```python
from build123d import *

# Parameters (mm, degrees)
PAD_DEPTH       = 6
SKETCH001_R     = 2
POCKET_DEPTH    = 8
POCKET001_DEPTH = 7


with BuildPart() as part:
    # Sketch → Pad (new body)
    with BuildSketch(Plane.XY):
        Polygon((1, 94.8), (7, 94.8), (7, 10), (8, 10), (8, 0), (0, 0), (0, 10), (1, 10), align=None)
    extrude(amount=PAD_DEPTH)

    # Sketch001 (on Face10 of Pad) → Pocket (cut)
    with BuildSketch(Plane.XY.offset(6)):
        with Locations((4, 4.995998)):
            Circle(SKETCH001_R)
    extrude(amount=-POCKET_DEPTH, mode=Mode.SUBTRACT)

    # Sketch002 (on Face5 of Pocket) → Pocket001 (cut)
    with BuildSketch(Plane.XY.offset(6)):
        with BuildLine():
            ThreePointArc((0, 1), (0.292893, 0.292893), (1, 0))
            Line((0, 0), (1, 0))
            Line((0, 1), (0, 0))
        make_face()
        with BuildLine():
            ThreePointArc((1, 10), (0.292893, 9.707107), (0, 9))
            Line((0, 9), (0, 10))
            Line((0, 10), (1, 10))
        make_face()
        with BuildLine():
            ThreePointArc((8, 9), (7.707107, 9.707107), (7, 10))
            Line((7, 10), (8, 10))
            Line((8, 10), (8, 9))
        make_face()
        with BuildLine():
            ThreePointArc((7, 0), (7.707107, 0.292893), (8, 1))
            Line((8, 0), (8, 1))
            Line((7, 0), (8, 0))
        make_face()
    extrude(amount=-POCKET001_DEPTH, mode=Mode.SUBTRACT)


solid = part.part
```
Verification items for the finished model (mm, model axes). A direction names the side the tool comes from. Round coordinates to 2 decimals unless told otherwise and drop trailing zeros. Order: outer loops, then holes, each group sorted by start corner. A loop starts at its lowest first (then second) coordinate and runs counter-clockwise, first axis right, second up. Notation, with made-up numbers: (51.25, -19) -> (98.25, -19) arc R18 ccw to (98.25, 15) -> close; hole circle Ø7 at (-7.5, 24.25). An arc over 180 degrees is marked (long way). Put each result on its own line as item: value. Start each with the question number.
(1) Material ranges on line 1 along Y through (x, z) = (3.75, 2.6); line 2 along X through (y, z) = (72.5, 2.7); line 3 along Y through (x, z) = (5.5, 5.65), recorded low to high.
(2) Tool access check on faces 1 (the face through (7, 53, 3)), 2 (the face through (1, 52, 3)), 3 (the face through (4, 48, 0)). Record the directions out of +Z, -Z, +X, -X, +Y, -Y that give a thin tool (end or side, any length) a straight path to the whole face; none if there is none.
(3) Section check B-B (z = 3.05). Enter the section's corners in (x, y), then the cut area to 3 significant figures.
(4) Section check C-C (y = 77.5). Enter the section's corners in (x, z).
(5) Section check A-A (x = 4). Enter the section's corners in (y, z), then the cut area to 3 significant figures.
(6) Depth check by flat-ended pin: pin 1 Ø1.8 at (y, z) = (32, 4.5) entering from +X; pin 2 Ø3 at (x, y) = (3.5, 73) entering from -Z. Enter the tip coordinate at first touch or a pass-through.
Completed:
1. line 1: y = 0 to 3.01, 6.98 to 94.8
1. line 2: x = 1 to 7
1. line 3: y = 0 to 3.67, 6.32 to 94.8
2. face 1: +Z, -Z, +X, +Y
2. face 2: +Z, -Z, -X, +Y
2. face 3: -Z, +X, -X, +Y, -Y
3. outline: (0, 1) arc R1 ccw to (1, 0) -> (7, 0) arc R1 ccw to (8, 1) -> (8, 9) arc R1 ccw to (7, 10) -> (7, 94.8) -> (1, 94.8) -> (1, 10) arc R1 ccw to (0, 9) -> close; hole circle Ø4 at (4, 5)
3. area: 575 mm2
4. outline: (1, 0) -> (7, 0) -> (7, 6) -> (1, 6) -> close
5. outline: (0, 0) -> (3, 0) -> (3, 6) -> (0, 6) -> close; (7, 0) -> (94.8, 0) -> (94.8, 6) -> (7, 6) -> close
5. area: 545 mm2
6. pin 1: stops at x = 7
6. pin 2: stops at z = 0
